from build123d import *

# Parameters (mm, degrees)
SKETCH1_W            = 52.99786638
SKETCH1_H            = 50.8
BOSS_EXTRUDE1_DEPTH  = 2.54
SKETCH2_R            = 1.27
CUT_EXTRUDE1_DEPTH   = 37.794090017
LPATTERN1_COUNT      = 2
LPATTERN1_PITCH      = 33.02
LPATTERN1_COUNT_DIR2 = 2
LPATTERN1_PITCH_DIR2 = 33.02
SKETCH3_R            = 13.335
SKETCH3_R_2          = 9.525
BOSS_EXTRUDE2_DEPTH  = 38.1
SKETCH4_R            = 1.27
CUT_EXTRUDE2_DEPTH   = 7.62
SKETCH5_R            = 1.27
CUT_EXTRUDE3_DEPTH   = 7.62


with BuildPart() as part:
    # Sketch1 → Boss-Extrude1 (new body)
    with BuildSketch(Plane(origin=(0, 0, 0), x_dir=(1, 0, 0), z_dir=(0, 1, 0))):
        Rectangle(SKETCH1_W, SKETCH1_H)
    extrude(amount=BOSS_EXTRUDE1_DEPTH)

    # Sketch2 → Cut-Extrude1 (cut, through all)
    with BuildSketch(Plane.XZ):
        with Locations(Location((-17.60893319, 16.51, 0), (0, 0, 270))):
            Circle(SKETCH2_R)
    cut_extrude1 = extrude(amount=-CUT_EXTRUDE1_DEPTH, mode=Mode.SUBTRACT)

    # LPattern1: Cut-Extrude1 2 × 2
    with Locations(*[(i * LPATTERN1_PITCH, 0, -j * LPATTERN1_PITCH_DIR2) for i in range(LPATTERN1_COUNT) for j in range(LPATTERN1_COUNT_DIR2) if (i, j) != (0, 0)]):
        add(cut_extrude1, mode=Mode.SUBTRACT)

    # Sketch3 → Boss-Extrude2 (add)
    with BuildSketch(Plane.XZ):
        with Locations(Location((0, 0, 0), (0, 0, 90))):
            Circle(SKETCH3_R)
        with Locations(Location((0, 0, 0), (0, 0, 90))):
            Circle(SKETCH3_R_2, mode=Mode.SUBTRACT)
    extrude(amount=BOSS_EXTRUDE2_DEPTH)

    # Sketch4 → Cut-Extrude2 (cut)
    with BuildSketch(Plane.XY.offset(13.335)):
        with Locations(Location((0, -20.78376556, 0), (0, 0, 270))):
            Circle(SKETCH4_R)
    extrude(amount=-CUT_EXTRUDE2_DEPTH, mode=Mode.SUBTRACT)

    # Sketch5 → Cut-Extrude3 (cut)
    with BuildSketch(Plane(origin=(13.335, 0, 0), x_dir=(0, 0, -1), z_dir=(1, 0, 0))):
        with Locations((0, -29.639158728)):
            Circle(SKETCH5_R)
    extrude(amount=-CUT_EXTRUDE3_DEPTH, mode=Mode.SUBTRACT)


solid = part.part
Geometry: final body of the model. Coordinates: model frame, mm. A direction names the side the tool comes from. Round coordinates to 2 decimals unless told otherwise and drop trailing zeros. Loops run counter-clockwise (first coordinate to the right, second up) from the corner with the lowest first, then second, coordinate; pieces in that order, holes last. Notation, with made-up numbers: (-2.75, 65) - (37.25, 65) arc R17 cw to (37.25, 93) - close; hole circle Ø2 at (86, 52). An arc over 180 degrees is marked (long way). Write each question's results on one line, items separated by ' | '. Start each with the question number.
1) Cut plane B-B on x = 0. Return loops of the section in (y, z) (3 decimals), then the cut area to 3 significant figures.
2) Access query for faces 1 (the face through (11.413, -30.879, 0.275)), 2 (the face through (5.796, -18.783, -7.559)), 3 (the face through (0.056, -19.515, 11.415)), 4 (the face through (-16.35, 1.25, -16.34)). Directions: +Z, -Z, +X, -X, +Y, -Y. A direction counts if a zero-diameter tool reaches every point of the face in a straight line with its end or side. Return the directions, or none.
3) First-contact query: P1, Ø6, axis at y = -4, z = 7.5, coming from the -X side; P2, Ø17, axis at x = 0, z = 0, coming from the -Y side; P3, Ø4, axis at y = -29.64, z = 0, coming from the +X side (3 decimals); P4, Ø12, axis at x = 7.5, y = -4.5, coming from the +Z side. Flat tips, straight axial feed; report the tip coordinate or a pass-through.
4) Mould query, pull axis X, two halves, no side actions, for faces 5 (the face through (-13.22, -18.78, -1.74)), 6 (the face through (0, 2.54, 0)), 7 (the face through (0, 0, 0)). Classes: released by +X, released by -X, zero draft, split by the parting line, or undercut.
5) Cut plane C-C on z = 0. Return loops of the section in (x, y) (3 decimals).
6) Cut plane A-A on z = 16.51. Return loops of the section in (x, y).
7) Cut plane D-D on y = -10.5. Return loops of the section in (x, z) (3 decimals).
8) Line query: probe 1 along X at (y, z) = (0.85, -16.51); probe 2 along Y at (x, z) = (11, 0); probe 3 along Z at (x, y) = (-0.5, -27). Output: solid intervals per line, ascending. Write a range as [from, to].
Verdict:
1) outline: (-38.1, -13.335) - (0, -13.335) - (0, -25.4) - (2.54, -25.4) - (2.54, 25.4) - (0, 25.4) - (0, 13.335) - (-19.514, 13.335) - (-19.514, 9.525) - (0, 9.525) - (0, -9.525) - (-38.1, -9.525) - close; (-38.1, 9.525) - (-22.054, 9.525) - (-22.054, 13.335) - (-38.1, 13.335) - close | area: 410 mm2
2) face 1: +X | face 2: -Y | face 3: +Z | face 4: +Y, -Y
3) P1: stops at x = -12.55 | P2: stops at y = 0 | P3: stops at x = 13.335 | P4: stops at z = 25.4
4) face 5: split by the parting line | face 6: zero draft | face 7: undercut
5) outline: (-26.499, 0) - (-13.335, 0) - (-13.335, -38.1) - (-9.525, -38.1) - (-9.525, 0) - (9.525, 0) - (9.525, -28.369) - (13.335, -28.369) - (13.335, 0) - (26.499, 0) - (26.499, 2.54) - (-26.499, 2.54) - close; (9.525, -38.1) - (13.335, -38.1) - (13.335, -30.909) - (9.525, -30.909) - close
6) outline: (-26.5, 0) - (-18.88, 0) - (-18.88, 2.54) - (-26.5, 2.54) - close; (-16.34, 0) - (14.14, 0) - (14.14, 2.54) - (-16.34, 2.54) - close; (16.68, 0) - (26.5, 0) - (26.5, 2.54) - (16.68, 2.54) - close
7) outline: circle Ø26.67 at (0, 0); hole circle Ø19.05 at (0, 0)
8) probe 1: x = [-26.5, -18.88], [-16.34, 14.14], [16.68, 26.5] | probe 2: y = [-38.1, -30.91], [-28.37, 2.54] | probe 3: z = [-13.33, -9.51], [9.51, 13.33]
